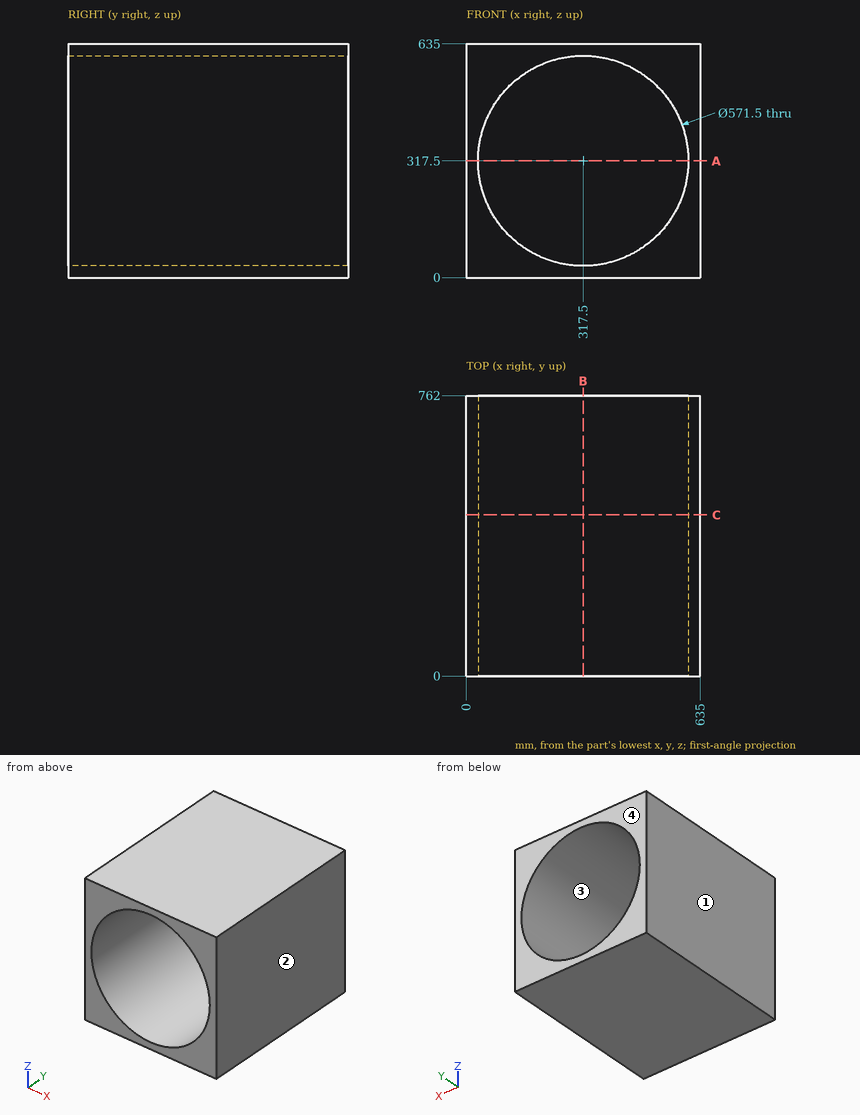
Source: three-view drawing plus pictorial views. Frame: mm from the lowest corner of the part. Round coordinates to 2 decimals unless told otherwise and drop trailing zeros. Loops run counter-clockwise (first coordinate to the right, second up) from the corner with the lowest first, then second, coordinate; pieces in that order, holes last.
Item 1: Section B-B, the plane x = 317.5. Output: boundary loops of the cut face in (y, z), plus the area to 3 significant figures.
Checked values:
outline: (0, 0) - (762, 0) - (762, 31.75) - (0, 31.75) - close; (0, 603.25) - (762, 603.25) - (762, 635) - (0, 635) - close
area: 48,400 mm2
Item 2: Line query: L1, parallel to X at y = 176, z = 317.5; L2, parallel to Z at x = 526, y = 568. Output: solid intervals per line, ascending.
Checked values:
L1: x = 0 to 31.75, 603.25 to 635
L2: z = 0 to 122.1, 512.9 to 635
Item 3: Section C-C, the plane y = 438. Output: boundary loops of the cut face in (x, z), plus the area to 3 significant figures.
Checked values:
outline: (0, 0) - (635, 0) - (635, 635) - (0, 635) - close; hole circle Ø571.5 at (317.5, 317.5)
area: 147,000 mm2
Item 4: Mould query, pull axis X, two halves, no side actions, for the marked faces 1, 2, 3 and 4. Classes: released by +X, released by -X, zero draft, split by the parting line, or undercut.
Checked values:
face 1: released by -X
face 2: released by +X
face 3: undercut
face 4: zero draft
Item 5: Section A-A, the plane z = 317.5. Output: boundary loops of the cut face in (x, y).
Checked values:
outline: (0, 0) - (31.75, 0) - (31.75, 762) - (0, 762) - close; (603.25, 0) - (635, 0) - (635, 762) - (603.25, 762) - close
